Part model, mm, in its own coordinate system. Round coordinates to 2 decimals unless told otherwise and drop trailing zeros. Answer as a JSON object with one key per item and string values. Group by question number.
1. Drill centre lines: line 1 (Y direction, x = 800, z = 1084); line 2 (Y direction, x = 12, z = 1078); line 3 (X direction, y = -445, z = 1072). Where is each one in solid material? Low to high. Write a range as from..to.
2. Band-saw the part on A-A, the plane z = 513. Count the separate pieces of the cut face and the enclosed holes in it, plus the area to 3 significant figures.
3. Two-plate mould, pull along X, no slides. Class faces 1 (the face through (1854.2, -10, 809)), 2 (the face through (1060, -190, 0)), 3 (the face through (0, -10, 809)), 4 (the face through (812.8, -600, 809)): +X half, -X half, draft (parallel to the pull), parting line (faces both ways), or undercut.
4. Drop flat-ended pins along their axis: pin 1 (20.5 mm diameter, centred on x = 798.5, y = -280.5, fed in from -Z); pin 2 (3.5 mm diameter, centred on y = -424.5, z = 1046.5, fed in from +X); pin 3 (4 mm diameter, centred on x = 1132.5, z = 636, fed in from -Y); pin 4 (3.5 mm diameter, centred on x = 1463.5, y = -425.5, fed in from -Z). Give the stop position or say it passes through.
from build123d import *

# Parameters (mm, degrees)
F0_W      = 25.4
F0_H      = 25.4
F1_DEPTH  = 609.6
F2_W      = 25.4
F2_H      = 25.4
F3_DEPTH  = 1854.2
F4_W      = 25.4
F4_H      = 25.4
F5_DEPTH  = 812.8
F6_W      = 25.4
F6_H      = 25.4
F7_DEPTH  = 1625.6
F8_W      = 25.4
F8_H      = 25.4
F9_DEPTH  = 1041.4
F10_W     = 1010.92
F10_H     = 1615.44
F11_DEPTH = 3.048
F12_W     = 1010.92
F12_H     = 1615.44
F13_DEPTH = 3.048
F14_R     = 6.35
F15_DEPTH = 1600.2


with BuildPart() as f1:
    # F0 (on Front) → F1 (new body)
    with BuildSketch(Plane.XZ):
        with Locations((12.7, 12.7)):
            Rectangle(F0_W, F0_H)
        with Locations((12.7, 546.1)):
            Rectangle(F0_W, F0_H)
        with Locations((12.7, 1079.5)):
            Rectangle(F0_W, F0_H)
        with Locations((12.7, 1612.9)):
            Rectangle(F0_W, F0_H)
        with Locations((800.1, 1612.9)):
            Rectangle(F0_W, F0_H)
        with Locations((800.1, 1079.5)):
            Rectangle(F0_W, F0_H)
        with Locations((800.1, 546.1)):
            Rectangle(F0_W, F0_H)
        with Locations((800.1, 12.7)):
            Rectangle(F0_W, F0_H)
        with Locations((1841.5, 1612.9)):
            Rectangle(F0_W, F0_H)
        with Locations((1841.5, 12.7)):
            Rectangle(F0_W, F0_H)
    extrude(amount=F1_DEPTH)

    # F2 (on Right) → F3 (join, through all)
    with BuildSketch(Plane.YZ):
        with Locations((-596.9, 1612.9)):
            Rectangle(F2_W, F2_H)
        with Locations((-12.7, 1612.9)):
            Rectangle(F2_W, F2_H)
        with Locations((-596.9, 12.7)):
            Rectangle(F2_W, F2_H)
        with Locations((-12.7, 12.7)):
            Rectangle(F2_W, F2_H)
    extrude(amount=F3_DEPTH)

    # F4 (on Right) → F5 (join, through all)
    with BuildSketch(Plane.YZ):
        with Locations((-596.9, 546.1)):
            Rectangle(F4_W, F4_H)
        with Locations((-12.7, 546.1)):
            Rectangle(F4_W, F4_H)
        with Locations((-596.9, 1079.5)):
            Rectangle(F4_W, F4_H)
        with Locations((-12.7, 1079.5)):
            Rectangle(F4_W, F4_H)
    extrude(amount=F5_DEPTH)

    # F6 (on Top) → F7 (join, through all)
    with BuildSketch(Plane.XY):
        with Locations((12.7, -12.7)):
            Rectangle(F6_W, F6_H)
        with Locations((800.1, -12.7)):
            Rectangle(F6_W, F6_H)
        with Locations((12.7, -596.9)):
            Rectangle(F6_W, F6_H)
        with Locations((800.1, -596.9)):
            Rectangle(F6_W, F6_H)
        with Locations((1841.5, -596.9)):
            Rectangle(F6_W, F6_H)
        with Locations((1841.5, -12.7)):
            Rectangle(F6_W, F6_H)
    extrude(amount=F7_DEPTH)

    # F8 (on face) → F9 (join, through all)
    with BuildSketch(Plane.YZ.offset(812.8)):
        with Locations((-410.633333, 1612.9)):
            Rectangle(F8_W, F8_H)
        with Locations((-198.966667, 1612.9)):
            Rectangle(F8_W, F8_H)
        with Locations((-410.633333, 12.7)):
            Rectangle(F8_W, F8_H)
        with Locations((-198.966667, 12.7)):
            Rectangle(F8_W, F8_H)
    extrude(amount=F9_DEPTH)

    # F10 (on face) → F11 (join)
    with BuildSketch(Plane.XZ.offset(423.333333)):
        with Locations((1343.66, 812.8)):
            Rectangle(F10_W, F10_H)
    extrude(amount=F11_DEPTH)

    # F12 (on face) → F13 (join)
    with BuildSketch(Plane(origin=(0, -186.266667, 0), x_dir=(-1, 0, 0), z_dir=(0, 1, 0))):
        with Locations((-1343.66, 812.8)):
            Rectangle(F12_W, F12_H)
    extrude(amount=F13_DEPTH)

    # F14 (on face) → F15 (cut, through all)
    with BuildSketch(Plane.XY.offset(1625.6)):
        with Locations((12.7, -416.814)):
            Circle(F14_R)
        with Locations((800.1, -416.814)):
            Circle(F14_R)
        with Locations((800.1, -192.786)):
            Circle(F14_R)
        with Locations((12.7, -192.786)):
            Circle(F14_R)
    extrude(amount=-F15_DEPTH, mode=Mode.SUBTRACT)


solid = f1.part
Worked answers:
{
 "1": {"line 1": "y = -609.6..-423.16, -410.46..-199.14, -186.44..0", "line 2": "y = -609.6..-423.13, -410.5..-199.1, -186.47..0", "line 3": "x = 0..25.4, 787.4..812.8"},
 "2": {"separate pieces": "8", "enclosed holes": "0", "area": "10,000 mm^2"},
 "3": {"face 1": "+X half", "face 2": "draft", "face 3": "-X half", "face 4": "undercut"},
 "4": {"pin 1": "stops at z = 0", "pin 2": "stops at x = 1849.12", "pin 3": "stops at y = -426.38", "pin 4": "stops at z = 5.08"}
}
